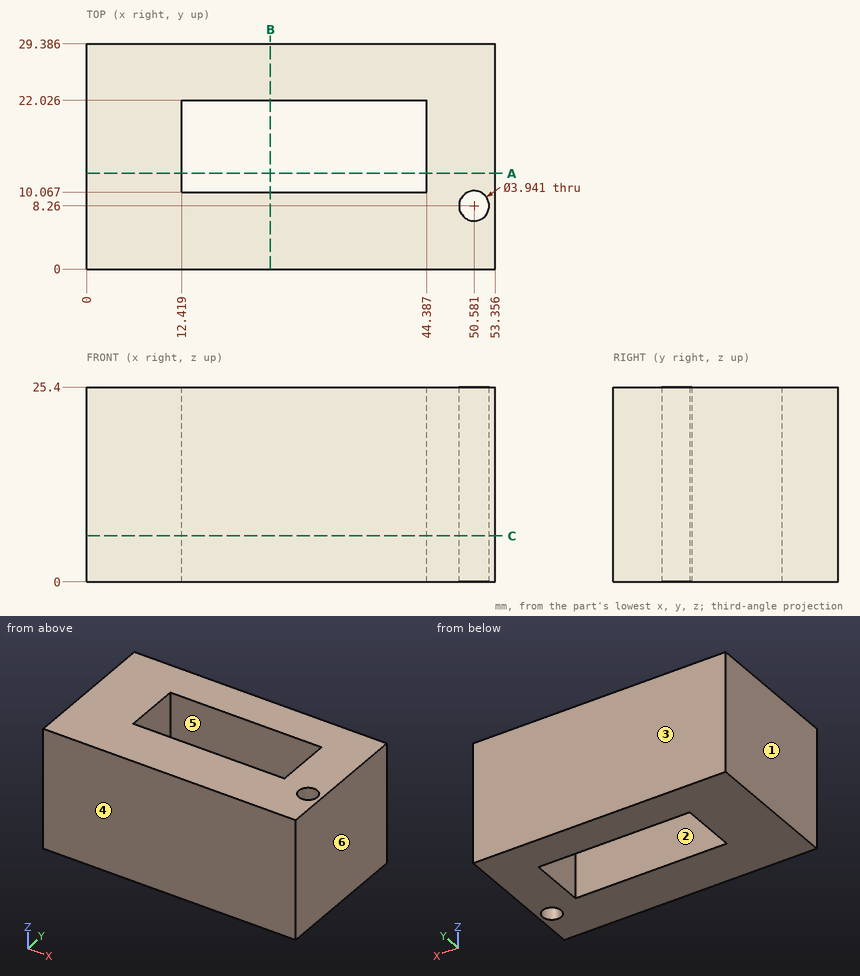
Input: dimensioned drawing with shaded views. Units: mm. Origin: part minimum x, y, z. A direction names the side the tool comes from. Round coordinates to 2 decimals unless told otherwise and drop trailing zeros. Write each loop counter-clockwise with the first axis right and the second up, starting at its lowest first coordinate (ties: lowest second). Pieces come first, ordered by that corner, then holes. Notation, with made-up numbers: (67, 84.5) -> (74, 84.5) arc R5 cw to (74, 88.5) -> close; hole circle Ø8 at (4.25, 36.5). An arc over 180 degrees is marked (long way). Use CSV: the item, a comma, the result in double quotes. Start each with the question number.
Q1. Section B-B (x = 24). Return loops of the section in (y, z) (1 decimal), plus the area to 3 significant figures.
Q2. Section C-C (z = 6). Return loops of the section in (x, y) (1 decimal).
Q3. Pull-direction query (Y, two-part tool) for the marked faces 3, 4, 5 and 6; classes: pulls with the +Y half, pulls with the -Y half, needs draft (parallel to the pull), parting line crosses it, or undercut.
Q4. Line query: L1, parallel to X at y = 17.75, z = 17 (1 decimal); L2, parallel to Y at x = 38, z = 9 (1 decimal); L3, parallel to Y at x = 49.5, z = 21.25 (1 decimal). Output: solid intervals per line, ascending.
Q5. Section A-A (y = 12.5). Return loops of the section in (x, z) (1 decimal).
Q6. Reachability of the marked faces 1 and 2 from +Z, -Z, +X, -X, +Y, -Y: full face, straight path, thin tool, end or side. Return the list, or none.
Result sheet:
1,outline,"(0, 0) -> (10.1, 0) -> (10.1, 25.4) -> (0, 25.4) -> close; (22, 0) -> (29.4, 0) -> (29.4, 25.4) -> (22, 25.4) -> close"
1,area,"443 mm²"
2,outline,"(0, 0) -> (53.4, 0) -> (53.4, 29.4) -> (0, 29.4) -> close; hole (12.4, 10.1) -> (44.4, 10.1) -> (44.4, 22) -> (12.4, 22) -> close; hole circle Ø3.9 at (50.6, 8.3)"
3,face 3,"pulls with the +Y half"
3,face 4,"pulls with the -Y half"
3,face 5,"undercut"
3,face 6,"needs draft"
4,L1,"0 to 12.4, 44.4 to 53.4"
4,L2,"0 to 10.1, 22 to 29.4"
4,L3,"0 to 6.6, 9.9 to 29.4"
5,outline,"(0, 0) -> (12.4, 0) -> (12.4, 25.4) -> (0, 25.4) -> close; (44.4, 0) -> (53.4, 0) -> (53.4, 25.4) -> (44.4, 25.4) -> close"
6,face 1,"+Z, -Z, -X, +Y, -Y"
6,face 2,"+Z, -Z"
